```python
from build123d import *

# Parameters (mm, degrees)
SKETCH1_R           = 30.48
BOSS_EXTRUDE1_DEPTH = 3.81
SKETCH2_R           = 1.9939
CUT_EXTRUDE1_DEPTH  = 44.273281595
CIRPATTERN1_COUNT   = 6


with BuildPart() as part:
    # Sketch1 → Boss-Extrude1 (new body)
    with BuildSketch(Plane(origin=(0, 0, 0), x_dir=(1, 0, 0), z_dir=(0, 1, 0))):
        with Locations(Location((0, 0, 0), (0, 0, 90))):
            Circle(SKETCH1_R)
    extrude(amount=BOSS_EXTRUDE1_DEPTH)

    # Sketch2 → Cut-Extrude1 (cut, through all)
    with BuildSketch(Plane(origin=(0, 3.81, 0), x_dir=(1, 0, 0), z_dir=(0, 1, 0))):
        with Locations(Location((0, -23.749, 0), (0, 0, 270))):
            Circle(SKETCH2_R)
    cut_extrude1 = extrude(amount=-CUT_EXTRUDE1_DEPTH, mode=Mode.SUBTRACT)

    # CirPattern1: Cut-Extrude1 ×6 about axis
    cirpattern1_axis = Axis((0, 0, 0), (0, 1, 0))
    for i in range(1, CIRPATTERN1_COUNT):
        add(cut_extrude1.rotate(cirpattern1_axis, i * 360 / CIRPATTERN1_COUNT), mode=Mode.SUBTRACT)


solid = part.part
```
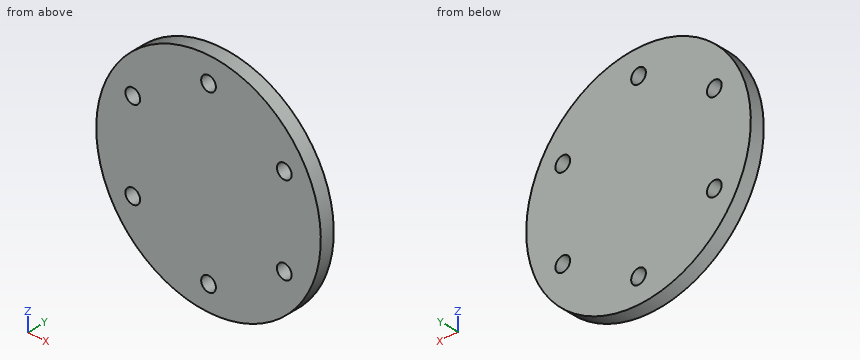
Check sheet for the modelled part. Datum: model origin and axes. Units: mm. Round coordinates to 2 decimals unless told otherwise and drop trailing zeros. Order: outer loops, then holes, each group sorted by start corner. A loop starts at its lowest first (then second) coordinate and runs counter-clockwise, first axis right, second up. Notation, with made-up numbers: (83.25, 54) -> (133.25, 54) arc R17 cw to (133.25, 70) -> close; hole circle Ø8 at (63.5, -13). An arc over 180 degrees is marked (long way). One line per item, written item: value. Start each with the question number.
Q1. Cross-section at A-A (x = 0). Record the boundary of the cut face in (y, z).
Q2. Gauge pin test, flat ends, axial feed: pin 1 Ø5 at (x, z) = (20.57, -11.87) entering from +Y; pin 2 Ø1.5 at (x, y) = (-15, 1.5) entering from +Z; pin 3 Ø3 at (x, z) = (0, 23.749) entering from +Y; pin 4 Ø2 at (y, z) = (3, 12) entering from +X. Record the tip position at first contact, or that the pin passes through.
Q3. Cross-section at D-D (x = -26). Record the boundary of the cut face in (y, z), and give its area (3 significant figures).
Q4. Cross-section at B-B (y = 2.8). Record the boundary of the cut face in (x, z), and give its area (3 significant figures).
Q5. Cross-section at C-C (z = -8.5). Record the boundary of the cut face in (x, y), and give its area (3 significant figures).
Q6. Thickness scan on line 1 (Z direction, x = 20.5, y = 3); line 2 (Z direction, x = 1.5, y = 0.5); line 3 (X direction, y = 2.2, z = -23). Record the ranges inside material, lowest first.
Completed:
1. outline: (0, -30.48) -> (3.81, -30.48) -> (3.81, -25.74) -> (0, -25.74) -> close; (0, -21.76) -> (3.81, -21.76) -> (3.81, 21.76) -> (0, 21.76) -> close; (0, 25.74) -> (3.81, 25.74) -> (3.81, 30.48) -> (0, 30.48) -> close
2. pin 1: stops at y = 3.81
2. pin 2: stops at z = 26.94
2. pin 3: passes through
2. pin 4: stops at x = 28.43
3. outline: (0, -15.91) -> (3.81, -15.91) -> (3.81, 15.91) -> (0, 15.91) -> close
3. area: 121 mm²
4. outline: circle Ø60.96 at (0, 0); hole circle Ø3.99 at (-20.57, -11.87); hole circle Ø3.99 at (-20.57, 11.87); hole circle Ø3.99 at (0, -23.75); hole circle Ø3.99 at (0, 23.75); hole circle Ø3.99 at (20.57, -11.87); hole circle Ø3.99 at (20.57, 11.87)
4. area: 2,840 mm²
5. outline: (-29.27, 0) -> (29.27, 0) -> (29.27, 3.81) -> (-29.27, 3.81) -> close
5. area: 223 mm²
6. line 1: z = -22.56 to -13.87, -9.88 to 9.88, 13.87 to 22.56
6. line 2: z = -30.44 to -25.06, -22.44 to 22.44, 25.06 to 30.44
6. line 3: x = -20 to -1.85, 1.85 to 20
